```python
from build123d import *

# Parameters (mm, degrees)
MODEL_R             = 1.3
BOSS_EXTRUDE1_DEPTH = 3


with BuildPart() as part:
    # Model → Boss-Extrude1 (new body)
    with BuildSketch(Plane.XY):
        with BuildLine():
            Line((48.62361742, 20.481068056), (39.12638258, 20.481068056))
            Line((39.12638258, 20.481068056), (39.12638258, 24.481068056))
            Line((39.12638258, 24.481068056), (40.37638258, 24.481068056))
            Line((40.37638258, 24.481068056), (40.37638258, 26.981068056))
            Line((40.37638258, 26.981068056), (39.12638258, 26.981068056))
            Line((39.12638258, 26.981068056), (39.12638258, 28.981068056))
            Line((39.12638258, 28.981068056), (36.12638258, 28.981068056))
            Line((36.12638258, 28.981068056), (36.12638258, 26.981068056))
            Line((36.12638258, 26.981068056), (34.87638258, 26.981068056))
            Line((34.87638258, 26.981068056), (34.87638258, 24.488530086))
            Line((34.87638258, 24.488530086), (36.12638258, 24.488530086))
            Line((36.12638258, 24.488530086), (36.12638258, 20.488530086))
            Line((36.12638258, 20.488530086), (32.37638258, 20.488530086))
            Line((32.37638258, 20.488530086), (32.37638258, 21.988530086))
            Line((32.37638258, 21.988530086), (29.37638258, 21.988530086))
            Line((29.37638258, 21.988530086), (29.37638258, 31.988530086))
            Line((29.37638258, 31.988530086), (32.37638258, 31.988530086))
            Line((32.37638258, 31.988530086), (32.37638258, 36.488530086))
            Line((32.37638258, 36.488530086), (35.395249636, 48.968623875))
            ThreePointArc((35.395249636, 48.968623875), (41.708225131, 53.498846113), (47.198169486, 48.000020412))
            Line((47.198169486, 48.000020412), (48.62361742, 32.814680991))
            Line((48.62361742, 32.814680991), (48.62361742, 20.481068056))
        make_face()
        with Locations((41.27638258, 47.488530086)):
            Circle(MODEL_R, mode=Mode.SUBTRACT)
    extrude(amount=BOSS_EXTRUDE1_DEPTH)


solid = part.part
```
Geometry: final body of the model. Coordinates: model frame, mm. A direction names the side the tool comes from. Coordinates: 2 decimals unless noted, no trailing zeros. Loops run counter-clockwise (first coordinate to the right, second up) from the corner with the lowest first, then second, coordinate; pieces in that order, holes last. Notation, with made-up numbers: (-3, 6.25) -> (32, 6.25) arc R22 cw to (32, 31.25) -> close; hole circle Ø8 at (84.25, 78). An arc over 180 degrees is marked (long way). Use a Markdown table: item, result. Add a question column.
(1) Section query B-B, the plane x = 41.5. Return loops of the section in (y, z).
(2) Pin query (flat end, axial travel): pin 1 Ø1.5 at (x, z) = (30.5, 1) entering from +Y; pin 2 Ø1.2 at (y, z) = (21, 1) entering from -X; pin 3 Ø1.5 at (x, z) = (45, 2) entering from +Y. Return the tip coordinate at first contact, or that it passes through.
(3) Section query D-D, the plane y = 44.5. Return loops of the section in (x, z), plus the area to 3 significant figures.
(4) Mould query, pull axis X, two halves, no side actions, for faces 1 (the flat face through (44, 20.481, 1)), 2 (the cylindrical face through (42.477, 46.991, 1.479)), 3 (the flat face through (32.376, 34, 1)). Classes: pulls with the +X half, pulls with the -X half, needs draft (parallel to the pull), parting line crosses it, or undercut.
(5) Access query for faces 4 (the flat face through (31, 21.989, 1)), 5 (the flat face through (40.376, 26, 1)), 6 (the flat face through (36.126, 23, 1)), 7 (the flat face through (31, 31.989, 1)). Directions: +Z, -Z, +X, -X, +Y, -Y. A direction counts if a zero-diameter tool reaches every point of the face in a straight line with its end or side. Return the directions, or none.
(6) Line query: line 1 along X through (y, z) = (23, 2.05); line 2 along X through (y, z) = (25, 1.1); line 3 along Y through (x, z) = (35.75, 1.8). Output: solid intervals per line, ascending.
(7) Section query C-C, the plane z = 0.7. Return loops of the section in (x, y).
(8) Section query A-A, the plane y = 25.5. Return loops of the section in (x, z).
Answer:
| question | item | result |
|---|---|---|
| 1 | outline | (20.48, 0) -> (46.21, 0) -> (46.21, 3) -> (20.48, 3) -> close; (48.77, 0) -> (53.51, 0) -> (53.51, 3) -> (48.77, 3) -> close |
| 2 | pin 1 | stops at y = 31.99 |
| 2 | pin 2 | stops at x = 32.38 |
| 2 | pin 3 | stops at y = 52.7 |
| 3 | outline | (34.31, 0) -> (47.53, 0) -> (47.53, 3) -> (34.31, 3) -> close |
| 3 | area | 39.6 mm^2 |
| 4 | face 1 | needs draft |
| 4 | face 2 | undercut |
| 4 | face 3 | pulls with the -X half |
| 5 | face 4 | +Z, -Z, -X, -Y |
| 5 | face 5 | +Z, -Z |
| 5 | face 6 | +Z, -Z, -Y |
| 5 | face 7 | +Z, -Z, -X, +Y |
| 6 | line 1 | x = 29.38 to 36.13, 39.13 to 48.62 |
| 6 | line 2 | x = 29.38 to 34.88, 40.38 to 48.62 |
| 6 | line 3 | y = 20.49 to 24.49, 26.98 to 49.99 |
| 7 | outline | (29.38, 21.99) -> (32.38, 21.99) -> (32.38, 20.49) -> (36.13, 20.49) -> (36.13, 24.49) -> (34.88, 24.49) -> (34.88, 26.98) -> (36.13, 26.98) -> (36.13, 28.98) -> (39.13, 28.98) -> (39.13, 26.98) -> (40.38, 26.98) -> (40.38, 24.48) -> (39.13, 24.48) -> (39.13, 20.48) -> (48.62, 20.48) -> (48.62, 32.81) -> (47.2, 48) arc R6 ccw to (35.4, 48.97) -> (32.38, 36.49) -> (32.38, 31.99) -> (29.38, 31.99) -> close; hole circle Ø2.6 at (41.28, 47.49) |
| 8 | outline | (29.38, 0) -> (34.88, 0) -> (34.88, 3) -> (29.38, 3) -> close; (40.38, 0) -> (48.62, 0) -> (48.62, 3) -> (40.38, 3) -> close |
